Check sheet for the modelled part. Datum: model origin and axes. Units: mm. A direction names the side the tool comes from. Coordinates: 2 decimals unless noted, no trailing zeros. Write each loop counter-clockwise with the first axis right and the second up, starting at its lowest first coordinate (ties: lowest second). Pieces come first, ordered by that corner, then holes. Notation, with made-up numbers: M 9.5,16.5 L 55.5,16.5 A18 ccw 55.5,42.5 Z; hole C -7,62 d1. An arc over 180 degrees is marked long. Answer as CSV lines item,"result". Start each with the question number.
1) Go/stop test with a flat-tipped pin: pin 1 Ø15.5 at (x, y) = (78, 34) entering from +Z. Record where the tip stops, or that it passes through.
2) Draft check along X on faces 4 (the flat face through (42, 64, 2)), 5 (the flat face through (110, 59, 4)), 6 (the flat face through (1.8, 86.9, 8)), 7 (the flat face through (0, 59, 4)). Enter one of: +X half, -X half, draft (parallel to the pull), parting line (faces both ways), or undercut.
3) Section check B-B (x = 38). Record the cut outline in (y, z).
4) Material ranges on L1, parallel to X at y = 18.5, z = 1.4; L2, parallel to Y at x = 78, z = 2.45; L3, parallel to Y at x = 32, z = 1.1, recorded low to high. Write a range as [from, to].
5) Access from +Z, -Z, +X, -X, +Y, -Y to the whole of each face (thin tool, end or side, straight path). Record for faces 1 (the flat face through (54, 0, 4)), 2 (the flat face through (22, 93, 2)), 3 (the flat face through (2, 59, 6)).
6) Section check C-C (y = 18.5). Record the cut outline in (x, z).
7) Section check D-D (z = 6.25). Record the cut outline in (x, y).
8) Section check A-A (y = 70). Record the cut outline in (x, z).
from build123d import *

# Parameters (mm, degrees)
SKETCH_W        = 110
SKETCH_H        = 120
SKETCH_R        = 2.5
PAD_DEPTH       = 8
SKETCH001_W     = 106
SKETCH001_H     = 116
POCKET_DEPTH    = 4
SKETCH002_R     = 11.5
SKETCH002_R_2   = 6
SKETCH002_W     = 12
SKETCH002_H     = 29
POCKET001_DEPTH = 8.001


with BuildPart() as part:
    # Sketch → Pad (new body)
    with BuildSketch(Plane.XY):
        with Locations((55, 60)):
            Rectangle(SKETCH_W, SKETCH_H)
        with Locations((32, 101.5)):
            Circle(SKETCH_R, mode=Mode.SUBTRACT)
        with Locations((78, 101.5)):
            Circle(SKETCH_R, mode=Mode.SUBTRACT)
        with Locations((32, 18.5)):
            Circle(SKETCH_R, mode=Mode.SUBTRACT)
        with Locations((78, 18.5)):
            Circle(SKETCH_R, mode=Mode.SUBTRACT)
    extrude(amount=PAD_DEPTH)

    # Sketch001 → Pocket (cut)
    with BuildSketch(Plane.XY.offset(8)):
        with Locations((55, 60)):
            Rectangle(SKETCH001_W, SKETCH001_H)
    extrude(amount=-POCKET_DEPTH, mode=Mode.SUBTRACT)

    # Sketch002 → Pocket001 (cut, through all)
    with BuildSketch(Plane(origin=(0, 0, 0), x_dir=(1, 0, 0), z_dir=(0, 0, -1))):
        with Locations((78, -70)):
            Circle(SKETCH002_R)
        with Locations((78, -34)):
            Circle(SKETCH002_R_2)
        with Locations((22, -41.5)):
            Rectangle(SKETCH002_W, SKETCH002_H)
        with Locations((42, -41.5)):
            Rectangle(SKETCH002_W, SKETCH002_H)
        with Locations((22, -78.5)):
            Rectangle(SKETCH002_W, SKETCH002_H)
        with Locations((42, -78.5)):
            Rectangle(SKETCH002_W, SKETCH002_H)
    extrude(amount=-POCKET001_DEPTH, mode=Mode.SUBTRACT)


solid = part.part
Results found:
1,pin 1,"stops at z = 4"
2,face 4,"undercut"
2,face 5,"+X half"
2,face 6,"draft"
2,face 7,"-X half"
3,outline,"M 0,0 L 27,0 L 27,4 L 2,4 L 2,8 L 0,8 Z; M 56,0 L 64,0 L 64,4 L 56,4 Z; M 93,0 L 120,0 L 120,8 L 118,8 L 118,4 L 93,4 Z"
4,L1,"x = [0, 29.5], [34.5, 75.5], [80.5, 110]"
4,L2,"y = [0, 16], [21, 28], [40, 58.5], [81.5, 99], [104, 120]"
4,L3,"y = [0, 16], [21, 99], [104, 120]"
5,face 1,"+Z, -Z, +X, -X, -Y"
5,face 2,"+Z, -Z"
5,face 3,"+Z"
6,outline,"M 0,0 L 29.5,0 L 29.5,4 L 2,4 L 2,8 L 0,8 Z; M 34.5,0 L 75.5,0 L 75.5,4 L 34.5,4 Z; M 80.5,0 L 110,0 L 110,8 L 108,8 L 108,4 L 80.5,4 Z"
7,outline,"M 0,0 L 110,0 L 110,120 L 0,120 Z; hole M 2,2 L 108,2 L 108,118 L 2,118 Z"
8,outline,"M 0,0 L 16,0 L 16,4 L 2,4 L 2,8 L 0,8 Z; M 28,0 L 36,0 L 36,4 L 28,4 Z; M 48,0 L 66.5,0 L 66.5,4 L 48,4 Z; M 89.5,0 L 110,0 L 110,8 L 108,8 L 108,4 L 89.5,4 Z"
